Here's how the part is built. I have some questions about the finished solid (model axes, mm). Face numbers are marked on the shaded views. Give positions to 0.01 mm unless a question says otherwise; leave off trailing zeros. Loops run counter-clockwise (first coordinate to the right, second up) from the corner with the lowest first, then second, coordinate; pieces in that order, holes last. Notation, with made-up numbers: (49.25, 73) -> (105.25, 73) arc R30 cw to (105.25, 95) -> close; hole circle Ø9 at (54.25, 20). An arc over 180 degrees is marked (long way). Answer in a Markdown table with one row per item. Add a question column.
Item 1: If we section it at A-A (y = 35): Write out the boundary of the cut face in (x, z).
Item 2: If we section it at B-B (x = -55): Write out the boundary of the cut face in (y, z), then the cut area to 3 significant figures.
Item 3: If we section it at C-C (z = -20.5): Write out the boundary of the cut face in (x, y).
Item 4: If I drill on line 1 (X direction, y = 35.5, z = -29); line 2 (Z direction, x = -14, y = -36), over which ranges is the centre line in solid material (lowest first)?
Item 5: If we section it at D-D (x = 48): Write out the boundary of the cut face in (y, z), then the cut area to 3 significant figures.
Item 6: For P1, Ø1, axis at x = -28, y = -27, coming from the -Z side, with a flat end and sliding along its axis, tell me the tip position at first contact or that it passes through.
Item 7: We'd pull the mould along Y, two halves only. Please class the marked faces 1 and 2: released by +Y, released by -Y, zero draft, split by the parting line, or undercut.
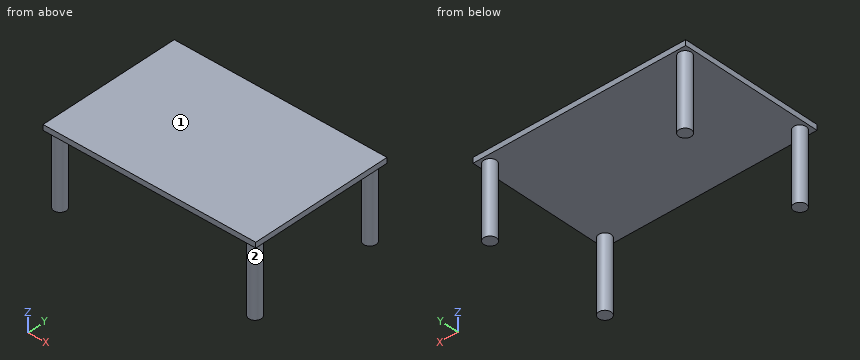
Autodesk Inventor part; units mm, degrees
ref_plane "YZ Plane" through (0, 0, 0) normal (1, 0, 0) x (0, 1, 0)
ref_plane "XZ Plane" through (0, 0, 0) normal (0, 1, 0) x (-1, 0, 0)
ref_plane "XY Plane" through (0, 0, 0) normal (0, 0, 1) x (1, 0, 0)
sketch "Sketch1" plane through (0, 0, 0) normal (0, 0, 1) x (1, 0, 0)
  line L0 (-50, -30) -> (50, -30) construction
  line L1 (50, -30) -> (50, 30) construction
  line L2 (50, 30) -> (-50, 30) construction
  line L3 (-50, 30) -> (-50, -30) construction
  line L4 (-50, -30) -> (50, 30) construction
  line L5 (50, -30) -> (-50, 30) construction
  line L6 (-60, -40) -> (60, -40)
  line L7 (60, -40) -> (60, 40)
  line L8 (60, 40) -> (-60, 40)
  line L9 (-60, 40) -> (-60, -40)
  line L10 (-60, -40) -> (60, 40)
  line L11 (60, -40) -> (-60, 40)
  point P0 (0, 0)
  dimension "d0" = 60
  dimension "d1" = 100
  dimension "d2" = 10
  dimension "d3" = 10
extrude "Extrusion1" add sketch "Sketch1" along normal blind 3
sketch "Sketch2" plane through (0, 0, 0) normal (0, 0, -1) x (-1, 0, 0)
  line L0 (50, -30) -> (50, 30) construction
  line L1 (50, 30) -> (-50, 30) construction
  line L2 (-50, 30) -> (-50, -30) construction
  line L3 (-50, -30) -> (50, -30) construction
  line L4 (50, -30) -> (-50, 30) construction
  line L5 (50, 30) -> (-50, -30) construction
  line L6 (60, -40) -> (-60, -40) construction
  line L7 (-50, -30) -> (-60, -30) construction
  line L8 (-60, -30) -> (-60, -40) construction
  line L9 (-60, -40) -> (-50, -40) construction
  line L10 (-50, -40) -> (-50, -30) construction
  line L11 (-60, 40) -> (60, 40) construction
  line L12 (-50, 30) -> (-60, 30) construction
  line L13 (-60, 30) -> (-60, 40) construction
  line L14 (-60, 40) -> (-50, 40) construction
  line L15 (-50, 40) -> (-50, 30) construction
  line L16 (50, 30) -> (60, 30) construction
  line L17 (60, 30) -> (60, 40) construction
  line L18 (60, 40) -> (50, 40) construction
  line L19 (50, 40) -> (50, 30) construction
  line L20 (60, 40) -> (60, -40) construction
  line L21 (60, -40) -> (50, -40) construction
  line L22 (50, -40) -> (50, -30) construction
  line L23 (50, -30) -> (60, -30) construction
  line L24 (60, -30) -> (60, -40) construction
  circle A0 centre (-55, -35) radius 3.5
  circle A1 centre (-55, 35) radius 3.5
  circle A2 centre (55, -35) radius 3.5
  circle A3 centre (55, 35) radius 3.5
  line L25 (-55, -35) -> (55, -35) construction
  line L26 (55, -35) -> (55, 35) construction
  line L27 (55, 35) -> (-55, 35) construction
  line L28 (-55, 35) -> (-55, -35) construction
  line L29 (-55, -35) -> (55, 35) construction
  line L30 (55, -35) -> (-55, 35) construction
  line L31 (-60, -40) -> (-60, 40) construction
  point P0 (0, 0)
  dimension "d6" = 60
  dimension "d7" = 100
  dimension "d8" = 7
  dimension "d9" = 7
  dimension "d10" = 7
  dimension "d11" = 7
  dimension "d12" = 5
  dimension "d13" = 5
extrude "Extrusion2" add sketch "Sketch2" along normal blind 40
equation "\"d3\" = d2"
equation "\"d6\" = d0"
equation "\"d7\" = d1"
equation "\"d12\" = 0.5 * d2"
equation "\"d13\" = d12"
properties part number "table top"
Recorded:
| question | item | result |
|---|---|---|
| 1 | outline | (-60, 0) -> (-58.5, 0) -> (-58.5, -40) -> (-51.5, -40) -> (-51.5, 0) -> (51.5, 0) -> (51.5, -40) -> (58.5, -40) -> (58.5, 0) -> (60, 0) -> (60, 3) -> (-60, 3) -> close |
| 2 | outline | (-40, 0) -> (-38.5, 0) -> (-38.5, -40) -> (-31.5, -40) -> (-31.5, 0) -> (31.5, 0) -> (31.5, -40) -> (38.5, -40) -> (38.5, 0) -> (40, 0) -> (40, 3) -> (-40, 3) -> close |
| 2 | area | 800 mm^2 |
| 3 | outline | circle Ø7 at (-55, -35); circle Ø7 at (-55, 35); circle Ø7 at (55, -35); circle Ø7 at (55, 35) |
| 4 | line 1 | x = -58.46 to -51.54, 51.54 to 58.46 |
| 4 | line 2 | z = 0 to 3 |
| 5 | outline | (-40, 0) -> (40, 0) -> (40, 3) -> (-40, 3) -> close |
| 5 | area | 240 mm^2 |
| 6 | P1 | stops at z = 0 |
| 7 | face 1 | zero draft |
| 7 | face 2 | undercut |
